from build123d import *

# Parameters (mm, degrees)
F0_W     = 127
F0_H     = 119
F0_W_2   = 117
F0_H_2   = 23.75
F1_DEPTH = 25.4


# Not quite as in the source:
# - a feature of the source that left no trace in its solid (it failed there, or was rolled back) is left out


with BuildPart() as f1:
    # F0 (on Top) → F1 (new body)
    with BuildSketch(Plane.XY):
        Rectangle(F0_W, F0_H)
        Polygon((58.5, -54.5), (-58.5, -54.5), (-58.5, -30.75), (-58.5, -28.25), (-58.5, -25.75), (-58.5, -2), (58.5, -2), (58.5, -25.75), (58.5, -28.25), (58.5, -30.75), align=None, mode=Mode.SUBTRACT)
        with BuildLine():
            Line((-58.5, 32.3772868405), (-58.5, 54.5))
            Line((-58.5, 54.5), (-44.399074127, 54.5))
            Line((-44.399074127, 54.5), (-34.350925873, 54.5))
            ThreePointArc((-34.350925873, 54.5), (-38.9600636195, 49.3402742154), (-40.625, 42.625))
            ThreePointArc((-40.625, 42.625), (-46.5938326725, 32.3229219329), (-58.5, 32.3772868405))
        make_face(mode=Mode.SUBTRACT)
        with BuildLine():
            Line((-18.149074127, 30.75), (-44.399074127, 30.75))
            ThreePointArc((-44.399074127, 30.75), (-39.7899363805, 35.9097257846), (-38.125, 42.625))
            ThreePointArc((-38.125, 42.625), (-26.25, 54.5), (-14.375, 42.625))
            ThreePointArc((-14.375, 42.625), (-12.7100636195, 35.9097257846), (-8.100925873, 30.75))
            Line((-8.100925873, 30.75), (-18.149074127, 30.75))
        make_face(mode=Mode.SUBTRACT)
        with Locations((0, 13.875)):
            Rectangle(F0_W_2, F0_H_2, mode=Mode.SUBTRACT)
        with BuildLine():
            ThreePointArc((11.875, 42.625), (0, 30.75), (-11.875, 42.625))
            ThreePointArc((-11.875, 42.625), (-13.5399363805, 49.3402742154), (-18.149074127, 54.5))
            Line((-18.149074127, 54.5), (18.149074127, 54.5))
            ThreePointArc((18.149074127, 54.5), (13.5399363805, 49.3402742154), (11.875, 42.625))
        make_face(mode=Mode.SUBTRACT)
        with BuildLine():
            ThreePointArc((14.375, 42.625), (26.25, 54.5), (38.125, 42.625))
            ThreePointArc((38.125, 42.625), (39.7899363805, 35.9097257846), (44.399074127, 30.75))
            Line((44.399074127, 30.75), (8.100925873, 30.75))
            ThreePointArc((8.100925873, 30.75), (12.7100636195, 35.9097257846), (14.375, 42.625))
        make_face(mode=Mode.SUBTRACT)
        with BuildLine():
            Line((34.350925873, 54.5), (58.5, 54.5))
            Line((58.5, 54.5), (58.5, 32.3772868405))
            ThreePointArc((58.5, 32.3772868405), (46.5938326725, 32.3229219329), (40.625, 42.625))
            ThreePointArc((40.625, 42.625), (38.9600636195, 49.3402742154), (34.350925873, 54.5))
        make_face(mode=Mode.SUBTRACT)
    extrude(amount=F1_DEPTH)


solid = f1.part
Check sheet for the modelled part. Datum: model origin and axes. Units: mm. A direction names the side the tool comes from. Round coordinates to 2 decimals unless told otherwise and drop trailing zeros. Order: outer loops, then holes, each group sorted by start corner. A loop starts at its lowest first (then second) coordinate and runs counter-clockwise, first axis right, second up. Notation, with made-up numbers: M 32,25.25 L 82,25.25 A14 ccw 82,31.25 Z; hole C 68,65 d3. An arc over 180 degrees is marked long. One line per item, written item: value. Start each with the question number.
1. Section check C-C on x = 26.25. Enter the section's corners in (y, z).
2. Scan lines: line 1 along X through (y, z) = (-39.5, 18.75); line 2 along Y through (x, z) = (-17, 23); line 3 along Y through (x, z) = (33, 14.25). Record each from-to range of solid material in increasing order.
3. Section check B-B on y = -12.5. Enter the section's corners in (x, z), and give its area (3 significant figures).
4. Access from +Z, -Z, +X, -X, +Y, -Y to the whole of each face (thin tool, end or side, straight path). Record for faces 5 (the flat face through (63.5, -1, 13)), 6 (the flat face through (-1, 25.75, 13)).
5. Section check A-A on z = 20.75. Give the number of separate pieces and of enclosed holes in the cut face, and give its area (3 significant figures).
6. Release check for a two-part mould opening along Y. For faces 1 (the flat face through (-63.5, -1, 13)), 2 (the cylindrical face through (-46.443, 32.411, 12.522)), 3 (the flat face through (27, 30.75, 13)), 4 (the flat face through (-1, -59.5, 13)) record: released by +Y, released by -Y, zero draft, split by the parting line, or undercut.
7. Section check D-D on x = -36. Enter the section's corners in (y, z).
Results found:
1. outline: M -59.5,0 L -54.5,0 L -54.5,25.4 L -59.5,25.4 Z; M -2,0 L 2,0 L 2,25.4 L -2,25.4 Z; M 25.75,0 L 30.75,0 L 30.75,25.4 L 25.75,25.4 Z; M 54.5,0 L 59.5,0 L 59.5,25.4 L 54.5,25.4 Z
2. line 1: -63.5 to -58.5, 58.5 to 63.5
2. line 2: -59.5 to -54.5, -2 to 2, 25.75 to 30.75, 50.07 to 53.63, 54.5 to 59.5
2. line 3: -59.5 to -54.5, -2 to 2, 25.75 to 30.75, 52.4 to 59.5
3. outline: M -63.5,0 L -58.5,0 L -58.5,25.4 L -63.5,25.4 Z; M 58.5,0 L 63.5,0 L 63.5,25.4 L 58.5,25.4 Z
3. area: 254 mm^2
4. face 5: +Z, -Z, +X, +Y, -Y
4. face 6: +Z, -Z
5. separate pieces: 1
5. enclosed holes: 7
5. area: 3,720 mm^2
6. face 1: zero draft
6. face 2: undercut
6. face 3: undercut
6. face 4: released by -Y
7. outline: M -59.5,0 L -54.5,0 L -54.5,25.4 L -59.5,25.4 Z; M -2,0 L 2,0 L 2,25.4 L -2,25.4 Z; M 25.75,0 L 30.75,0 L 30.75,25.4 L 25.75,25.4 Z; M 49.4,0 L 53.19,0 L 53.19,25.4 L 49.4,25.4 Z; M 54.5,0 L 59.5,0 L 59.5,25.4 L 54.5,25.4 Z
